Model file for the job. Use its own axes, mm. Round coordinates to 2 decimals unless told otherwise and drop trailing zeros. Loops run counter-clockwise (first coordinate to the right, second up) from the corner with the lowest first, then second, coordinate; pieces in that order, holes last.
from build123d import *

# Parameters (mm, degrees)
SKETCH1_R           = 14.2875
BOSS_EXTRUDE1_DEPTH = 3.175
CUT_EXTRUDE1_REACH  = 5.175
SKETCH2_R           = 3.556
SKETCH2_R_2         = 3.175
CUT_EXTRUDE2_REACH  = 5.175
SKETCH3_R           = 2.667
CUT_EXTRUDE3_REACH  = 5.175
SKETCH4_R           = 2.667
CUT_EXTRUDE4_REACH  = 5.175
SKETCH6_R           = 14.2875


with BuildPart() as part:
    # Sketch1 → Boss-Extrude1 (new body)
    with BuildSketch(Plane(origin=(0, 0, 0), x_dir=(1, 0, 0), z_dir=(0, 1, 0))):
        with BuildLine():
            Line((-26.9875, 0), (-26.9875, -95.25))
            ThreePointArc((-26.9875, -95.25), (-25.127628061, -99.740128061), (-20.6375, -101.6))
            Line((-20.6375, -101.6), (423.8625, -101.6))
            ThreePointArc((423.8625, -101.6), (428.352628061, -99.740128061), (430.2125, -95.25))
            Line((430.2125, -95.25), (430.2125, 0))
            ThreePointArc((430.2125, 0), (403.225, 26.9875), (376.2375, 0))
            Line((376.2375, 0), (376.2375, -31.75))
            ThreePointArc((376.2375, -31.75), (374.377628061, -36.240128061), (369.8875, -38.1))
            Line((369.8875, -38.1), (33.3375, -38.1))
            ThreePointArc((33.3375, -38.1), (28.847371939, -36.240128061), (26.9875, -31.75))
            Line((26.9875, -31.75), (26.9875, 0))
            ThreePointArc((26.9875, 0), (0, 26.9875), (-26.9875, 0))
        make_face()
        Circle(SKETCH1_R, mode=Mode.SUBTRACT)
        with Locations((403.225, 0)):
            Circle(SKETCH1_R, mode=Mode.SUBTRACT)
    extrude(amount=BOSS_EXTRUDE1_DEPTH)

    # Sketch2 → Cut-Extrude1 (cut, up to next)
    with BuildSketch(Plane(origin=(0, 3.175, 0), x_dir=(1, 0, 0), z_dir=(0, 1, 0)), mode=Mode.PRIVATE) as cut_extrude1_sk1:
        with Locations((204.1525, -88.9)):
            Circle(SKETCH2_R)
    cut_extrude1_tool1 = extrude(cut_extrude1_sk1.sketch, amount=-CUT_EXTRUDE1_REACH, mode=Mode.PRIVATE) & part.part
    add(cut_extrude1_tool1.solids().sort_by_distance((204.1525, 3.175, 88.9))[0], mode=Mode.SUBTRACT)
    # Sketch2 → Cut-Extrude1 (cut, up to next)
    with BuildSketch(Plane(origin=(0, 3.175, 0), x_dir=(1, 0, 0), z_dir=(0, 1, 0)), mode=Mode.PRIVATE) as cut_extrude1_sk2:
        with Locations((199.0725, -53.34)):
            Circle(SKETCH2_R_2)
    cut_extrude1_tool2 = extrude(cut_extrude1_sk2.sketch, amount=-CUT_EXTRUDE1_REACH, mode=Mode.PRIVATE) & part.part
    add(cut_extrude1_tool2.solids().sort_by_distance((199.0725, 3.175, 53.34))[0], mode=Mode.SUBTRACT)

    # Sketch3 → Cut-Extrude2 (cut, up to next)
    with BuildSketch(Plane(origin=(0, 3.175, 0), x_dir=(1, 0, 0), z_dir=(0, 1, 0)), mode=Mode.PRIVATE) as cut_extrude2_sk1:
        with Locations((-15.779743521, -55.159030044)):
            Circle(SKETCH3_R)
    cut_extrude2_tool1 = extrude(cut_extrude2_sk1.sketch, amount=-CUT_EXTRUDE2_REACH, mode=Mode.PRIVATE) & part.part
    add(cut_extrude2_tool1.solids().sort_by_distance((-15.779744, 3.175, 55.15903))[0], mode=Mode.SUBTRACT)
    # Sketch3 → Cut-Extrude2 (cut, up to next)
    with BuildSketch(Plane(origin=(0, 3.175, 0), x_dir=(1, 0, 0), z_dir=(0, 1, 0)), mode=Mode.PRIVATE) as cut_extrude2_sk2:
        with Locations((419.004743521, -55.159030044)):
            Circle(SKETCH3_R)
    cut_extrude2_tool2 = extrude(cut_extrude2_sk2.sketch, amount=-CUT_EXTRUDE2_REACH, mode=Mode.PRIVATE) & part.part
    add(cut_extrude2_tool2.solids().sort_by_distance((419.004744, 3.175, 55.15903))[0], mode=Mode.SUBTRACT)
    # Sketch3 → Cut-Extrude2 (cut, up to next)
    with BuildSketch(Plane(origin=(0, 3.175, 0), x_dir=(1, 0, 0), z_dir=(0, 1, 0)), mode=Mode.PRIVATE) as cut_extrude2_sk3:
        with Locations((-15.779743521, -83.371493131)):
            Circle(SKETCH3_R)
    cut_extrude2_tool3 = extrude(cut_extrude2_sk3.sketch, amount=-CUT_EXTRUDE2_REACH, mode=Mode.PRIVATE) & part.part
    add(cut_extrude2_tool3.solids().sort_by_distance((-15.779744, 3.175, 83.371493))[0], mode=Mode.SUBTRACT)
    # Sketch3 → Cut-Extrude2 (cut, up to next)
    with BuildSketch(Plane(origin=(0, 3.175, 0), x_dir=(1, 0, 0), z_dir=(0, 1, 0)), mode=Mode.PRIVATE) as cut_extrude2_sk4:
        with Locations((419.004743521, -83.371493131)):
            Circle(SKETCH3_R)
    cut_extrude2_tool4 = extrude(cut_extrude2_sk4.sketch, amount=-CUT_EXTRUDE2_REACH, mode=Mode.PRIVATE) & part.part
    add(cut_extrude2_tool4.solids().sort_by_distance((419.004744, 3.175, 83.371493))[0], mode=Mode.SUBTRACT)

    # Sketch4 → Cut-Extrude3 (cut, up to next)
    with BuildSketch(Plane(origin=(0, 3.175, 0), x_dir=(1, 0, 0), z_dir=(0, 1, 0)), mode=Mode.PRIVATE) as cut_extrude3_sk1:
        with Locations((201.6125, -69.85)):
            Circle(SKETCH4_R)
    cut_extrude3_tool1 = extrude(cut_extrude3_sk1.sketch, amount=-CUT_EXTRUDE3_REACH, mode=Mode.PRIVATE) & part.part
    add(cut_extrude3_tool1.solids().sort_by_distance((201.6125, 3.175, 69.85))[0], mode=Mode.SUBTRACT)

    # Sketch6 → Cut-Extrude4 (cut, up to next)
    with BuildSketch(Plane(origin=(0, 3.175, 0), x_dir=(1, 0, 0), z_dir=(0, 1, 0)), mode=Mode.PRIVATE) as cut_extrude4_sk1:
        with Locations((11.501671414, -77.36717452)):
            Circle(SKETCH6_R)
    cut_extrude4_tool1 = extrude(cut_extrude4_sk1.sketch, amount=-CUT_EXTRUDE4_REACH, mode=Mode.PRIVATE) & part.part
    add(cut_extrude4_tool1.solids().sort_by_distance((11.501671, 3.175, 77.367175))[0], mode=Mode.SUBTRACT)
    # Sketch6 → Cut-Extrude4 (cut, up to next)
    with BuildSketch(Plane(origin=(0, 3.175, 0), x_dir=(1, 0, 0), z_dir=(0, 1, 0)), mode=Mode.PRIVATE) as cut_extrude4_sk2:
        with Locations((43.002904056, -58.635968615)):
            Circle(SKETCH6_R)
    cut_extrude4_tool2 = extrude(cut_extrude4_sk2.sketch, amount=-CUT_EXTRUDE4_REACH, mode=Mode.PRIVATE) & part.part
    add(cut_extrude4_tool2.solids().sort_by_distance((43.002904, 3.175, 58.635969))[0], mode=Mode.SUBTRACT)
    # Sketch6 → Cut-Extrude4 (cut, up to next)
    with BuildSketch(Plane(origin=(0, 3.175, 0), x_dir=(1, 0, 0), z_dir=(0, 1, 0)), mode=Mode.PRIVATE) as cut_extrude4_sk3:
        with Locations((75.001671414, -77.36717452)):
            Circle(SKETCH6_R)
    cut_extrude4_tool3 = extrude(cut_extrude4_sk3.sketch, amount=-CUT_EXTRUDE4_REACH, mode=Mode.PRIVATE) & part.part
    add(cut_extrude4_tool3.solids().sort_by_distance((75.001671, 3.175, 77.367175))[0], mode=Mode.SUBTRACT)
    # Sketch6 → Cut-Extrude4 (cut, up to next)
    with BuildSketch(Plane(origin=(0, 3.175, 0), x_dir=(1, 0, 0), z_dir=(0, 1, 0)), mode=Mode.PRIVATE) as cut_extrude4_sk4:
        with Locations((106.502904056, -58.635968615)):
            Circle(SKETCH6_R)
    cut_extrude4_tool4 = extrude(cut_extrude4_sk4.sketch, amount=-CUT_EXTRUDE4_REACH, mode=Mode.PRIVATE) & part.part
    add(cut_extrude4_tool4.solids().sort_by_distance((106.502904, 3.175, 58.635969))[0], mode=Mode.SUBTRACT)
    # Sketch6 → Cut-Extrude4 (cut, up to next)
    with BuildSketch(Plane(origin=(0, 3.175, 0), x_dir=(1, 0, 0), z_dir=(0, 1, 0)), mode=Mode.PRIVATE) as cut_extrude4_sk5:
        with Locations((138.501671414, -77.36717452)):
            Circle(SKETCH6_R)
    cut_extrude4_tool5 = extrude(cut_extrude4_sk5.sketch, amount=-CUT_EXTRUDE4_REACH, mode=Mode.PRIVATE) & part.part
    add(cut_extrude4_tool5.solids().sort_by_distance((138.501671, 3.175, 77.367175))[0], mode=Mode.SUBTRACT)
    # Sketch6 → Cut-Extrude4 (cut, up to next)
    with BuildSketch(Plane(origin=(0, 3.175, 0), x_dir=(1, 0, 0), z_dir=(0, 1, 0)), mode=Mode.PRIVATE) as cut_extrude4_sk6:
        with Locations((170.002904056, -58.635968615)):
            Circle(SKETCH6_R)
    cut_extrude4_tool6 = extrude(cut_extrude4_sk6.sketch, amount=-CUT_EXTRUDE4_REACH, mode=Mode.PRIVATE) & part.part
    add(cut_extrude4_tool6.solids().sort_by_distance((170.002904, 3.175, 58.635969))[0], mode=Mode.SUBTRACT)
    # Sketch6 → Cut-Extrude4 (cut, up to next)
    with BuildSketch(Plane(origin=(0, 3.175, 0), x_dir=(1, 0, 0), z_dir=(0, 1, 0)), mode=Mode.PRIVATE) as cut_extrude4_sk7:
        with Locations((233.222095944, -58.635968615)):
            Circle(SKETCH6_R)
    cut_extrude4_tool7 = extrude(cut_extrude4_sk7.sketch, amount=-CUT_EXTRUDE4_REACH, mode=Mode.PRIVATE) & part.part
    add(cut_extrude4_tool7.solids().sort_by_distance((233.222096, 3.175, 58.635969))[0], mode=Mode.SUBTRACT)
    # Sketch6 → Cut-Extrude4 (cut, up to next)
    with BuildSketch(Plane(origin=(0, 3.175, 0), x_dir=(1, 0, 0), z_dir=(0, 1, 0)), mode=Mode.PRIVATE) as cut_extrude4_sk8:
        with Locations((264.723328586, -77.36717452)):
            Circle(SKETCH6_R)
    cut_extrude4_tool8 = extrude(cut_extrude4_sk8.sketch, amount=-CUT_EXTRUDE4_REACH, mode=Mode.PRIVATE) & part.part
    add(cut_extrude4_tool8.solids().sort_by_distance((264.723329, 3.175, 77.367175))[0], mode=Mode.SUBTRACT)
    # Sketch6 → Cut-Extrude4 (cut, up to next)
    with BuildSketch(Plane(origin=(0, 3.175, 0), x_dir=(1, 0, 0), z_dir=(0, 1, 0)), mode=Mode.PRIVATE) as cut_extrude4_sk9:
        with Locations((296.722095944, -58.635968615)):
            Circle(SKETCH6_R)
    cut_extrude4_tool9 = extrude(cut_extrude4_sk9.sketch, amount=-CUT_EXTRUDE4_REACH, mode=Mode.PRIVATE) & part.part
    add(cut_extrude4_tool9.solids().sort_by_distance((296.722096, 3.175, 58.635969))[0], mode=Mode.SUBTRACT)
    # Sketch6 → Cut-Extrude4 (cut, up to next)
    with BuildSketch(Plane(origin=(0, 3.175, 0), x_dir=(1, 0, 0), z_dir=(0, 1, 0)), mode=Mode.PRIVATE) as cut_extrude4_sk10:
        with Locations((328.223328586, -77.36717452)):
            Circle(SKETCH6_R)
    cut_extrude4_tool10 = extrude(cut_extrude4_sk10.sketch, amount=-CUT_EXTRUDE4_REACH, mode=Mode.PRIVATE) & part.part
    add(cut_extrude4_tool10.solids().sort_by_distance((328.223329, 3.175, 77.367175))[0], mode=Mode.SUBTRACT)
    # Sketch6 → Cut-Extrude4 (cut, up to next)
    with BuildSketch(Plane(origin=(0, 3.175, 0), x_dir=(1, 0, 0), z_dir=(0, 1, 0)), mode=Mode.PRIVATE) as cut_extrude4_sk11:
        with Locations((360.222095944, -58.635968615)):
            Circle(SKETCH6_R)
    cut_extrude4_tool11 = extrude(cut_extrude4_sk11.sketch, amount=-CUT_EXTRUDE4_REACH, mode=Mode.PRIVATE) & part.part
    add(cut_extrude4_tool11.solids().sort_by_distance((360.222096, 3.175, 58.635969))[0], mode=Mode.SUBTRACT)
    # Sketch6 → Cut-Extrude4 (cut, up to next)
    with BuildSketch(Plane(origin=(0, 3.175, 0), x_dir=(1, 0, 0), z_dir=(0, 1, 0)), mode=Mode.PRIVATE) as cut_extrude4_sk12:
        with Locations((391.723328586, -77.36717452)):
            Circle(SKETCH6_R)
    cut_extrude4_tool12 = extrude(cut_extrude4_sk12.sketch, amount=-CUT_EXTRUDE4_REACH, mode=Mode.PRIVATE) & part.part
    add(cut_extrude4_tool12.solids().sort_by_distance((391.723329, 3.175, 77.367175))[0], mode=Mode.SUBTRACT)


solid = part.part
Q1. Pull direction Z, two halves, no side cores. Call faces 1 (the face through (176.6, 1.61, 71.31)), 2 (the face through (198, 0, 65)), 3 (the face through (373.42, 1.61, 64.11)), 4 (the face through (0.59, 1.57, -26.98)): pulls with the +Z half, pulls with the -Z half, needs draft (parallel to the pull), parting line crosses it, or undercut.
Q2. Slice it at A-A on x = 38. Give the cut face in (y, z) (3 decimals), plus the area to 3 significant figures.
Q3. Slice it at B-B on z = 7.5. Give the cut face in (x, y) (1 decimal).
Q4. Slice it at C-C on y = 2.65. State how many separate pieces and enclosed holes the cut face has, plus the area to 3 significant figures.
Q5. Flat gauge pin, fed straight in: P1, Ø1.5, axis at x = 90, y = 2, coming from the -Z side. Where does the tip first touch, or does it go through?
Q6. Probe line 1 (X direction, y = 1.35, z = 29); line 2 (X direction, y = 1.05, z = 11.5); line 3 (X direction, y = 2.2, z = 11). List the from-to ranges inside material, lowest first.
Reply:
1. face 1: undercut
1. face 2: needs draft
1. face 3: undercut
1. face 4: pulls with the -Z half
2. outline: (0, 38.1) - (3.175, 38.1) - (3.175, 45.253) - (0, 45.253) - close; (0, 72.019) - (3.175, 72.019) - (3.175, 101.6) - (0, 101.6) - close
2. area: 117 mm2
3. outline: (-27, 0) - (-12.2, 0) - (-12.2, 3.2) - (-27, 3.2) - close; (12.2, 0) - (27, 0) - (27, 3.2) - (12.2, 3.2) - close; (376.2, 0) - (391.1, 0) - (391.1, 3.2) - (376.2, 3.2) - close; (415.4, 0) - (430.2, 0) - (430.2, 3.2) - (415.4, 3.2) - close
4. separate pieces: 1
4. enclosed holes: 21
4. area: 26,300 mm2
5. P1: stops at z = 38.1
6. line 1: x = -26.99 to 26.99, 376.24 to 430.21
6. line 2: x = -26.99 to -8.48, 8.48 to 26.99, 376.24 to 394.75, 411.7 to 430.21
6. line 3: x = -26.99 to -9.12, 9.12 to 26.99, 376.24 to 394.11, 412.34 to 430.21
